from build123d import *

# Parameters (mm, degrees)
BOSS_EXTRUDE1_DEPTH = 2
BOSS_EXTRUDE2_DEPTH = 26
SKETCH2_W           = 20.4
SKETCH2_H           = 20.4
CUT_EXTRUDE1_DEPTH  = 30
CIRPATTERN1_COUNT   = 3
CUT_EXTRUDE2_DEPTH  = 104.592686872
SKETCH4_R           = 2
CUT_EXTRUDE3_DEPTH  = 10
BOSS_EXTRUDE4_START = 26
BOSS_EXTRUDE4_DEPTH = 10
SKETCH5_R           = 2
CUT_EXTRUDE4_DEPTH  = 10
CIRPATTERN2_COUNT   = 3


with BuildPart() as part:
    # Sketch1 → Boss-Extrude1 (new body)
    with BuildSketch(Plane(origin=(0, 0, 0), x_dir=(1, 0, 0), z_dir=(0, 1, 0))):
        Polygon((15, -25.980762114), (30, 0), (15, 25.980762114), (-15, 25.980762114), (-30, 0), (-15, -25.980762114), align=None)
    extrude(amount=BOSS_EXTRUDE1_DEPTH)

    # Sketch1<3> → Boss-Extrude2 (add)
    # profile 1 of 2: a face of its own
    with BuildSketch(Plane(origin=(0, 0, 0), x_dir=(1, 0, 0), z_dir=(0, 1, 0))):
        Polygon((-13, 72.494446501), (-41.141016151, 23.75277675), (-69.282032303, -24.988893001), (-56.282032303, -47.505553499), (0, -47.505553499), (56.282032303, -47.505553499), (69.282032303, -24.988893001), (41.141016151, 23.75277675), (13, 72.494446501), align=None)
        Polygon((-54.549981495, -44.505553499), (-65.817930688, -24.988893001), (-38.54293994, 22.25277675), (-11.267949192, 69.494446501), (11.267949192, 69.494446501), (38.54293994, 22.25277675), (65.817930688, -24.988893001), (54.549981495, -44.505553499), (0, -44.505553499), align=None, mode=Mode.SUBTRACT)
    # profile 2 of 2: a face of its own
    with BuildSketch(Plane(origin=(0, 0, 0), x_dir=(1, 0, 0), z_dir=(0, 1, 0))):
        Polygon((-65.817930688, -24.988893001), (-38.54293994, 22.25277675), (-11.267949192, 69.494446501), (11.267949192, 69.494446501), (38.54293994, 22.25277675), (65.817930688, -24.988893001), (54.549981495, -44.505553499), (0, -44.505553499), (-54.549981495, -44.505553499), align=None)
        Polygon((30, 0), (15, 25.980762114), (-15, 25.980762114), (-30, 0), (-15, -25.980762114), (15, -25.980762114), align=None, mode=Mode.SUBTRACT)
    extrude(amount=BOSS_EXTRUDE2_DEPTH)

    # Sketch2 → Cut-Extrude1 (cut)
    with BuildSketch(Plane(origin=(62.782032303, 0, 36.24722325), x_dir=(0.499999999999999, 0, -0.8660254037844394), z_dir=(0.8660254037844394, 0, 0.499999999999999))):
        with Locations((0, 13)):
            Rectangle(SKETCH2_W, SKETCH2_H)
    cut_extrude1 = extrude(amount=-CUT_EXTRUDE1_DEPTH, mode=Mode.SUBTRACT)

    # CirPattern1: Cut-Extrude1 ×3 about axis
    cirpattern1_axis = Axis((0, 0, 0), (0, 1, 0))
    for i in range(1, CIRPATTERN1_COUNT):
        add(cut_extrude1.rotate(cirpattern1_axis, i * 360 / CIRPATTERN1_COUNT), mode=Mode.SUBTRACT)

    # Sketch3 → Cut-Extrude2 (cut, through all)
    with BuildSketch(Plane(origin=(0, 26, 0), x_dir=(1, 0, 0), z_dir=(0, 1, 0))):
        Polygon((-5.063466521, -1.191342951), (-5.751288694, 0), (-2.875644347, 4.980762114), (-1.5, 4.980762114), (1.5, 4.980762114), (2.875644347, 4.980762114), (5.751288694, 0), (5.063466521, -1.191342951), (3.563466521, -3.789419162), (2.875644347, -4.980762114), (-2.875644347, -4.980762114), (-3.563466521, -3.789419162), align=None)
        Polygon((6.161542732, -5.289419162), (6.911542732, -3.990381057), (7.661542732, -2.691342951), (9.215390309, 0), (7.661542732, 2.691342951), (10.259618943, 4.191342951), (12.679491924, 0), (9.509618943, -5.490381057), (6.339745962, -10.980762114), (1.5, -10.980762114), (1.5, -7.980762114), (4.607695155, -7.980762114), align=None)
        Polygon((-6.339745962, 10.980762114), (0, 10.980762114), (6.339745962, 10.980762114), (8.759618943, 6.789419162), (6.161542732, 5.289419162), (4.607695155, 7.980762114), (1.5, 7.980762114), (0, 7.980762114), (-1.5, 7.980762114), (-4.607695155, 7.980762114), (-6.161542732, 5.289419162), (-8.759618943, 6.789419162), align=None)
        Polygon((-7.661542732, -2.691342951), (-6.911542732, -3.990381057), (-6.161542732, -5.289419162), (-4.607695155, -7.980762114), (-1.5, -7.980762114), (-1.5, -10.980762114), (-6.339745962, -10.980762114), (-9.509618943, -5.490381057), (-12.679491924, 0), (-10.259618943, 4.191342951), (-7.661542732, 2.691342951), (-9.215390309, 0), align=None)
        Polygon((-9.803847577, -16.980762114), (-13.955771366, -9.789419162), (-11.357695155, -8.289419162), (-8.07179677, -13.980762114), (8.07179677, -13.980762114), (11.357695155, -8.289419162), (13.955771366, -9.789419162), (9.803847577, -16.980762114), align=None)
        Polygon((19.607695155, 0), (15.455771366, -7.191342951), (12.857695155, -5.691342951), (16.143593539, 0), (8.07179677, 13.980762114), (1.5, 13.980762114), (1.5, 16.980762114), (9.803847577, 16.980762114), align=None)
        Polygon((-9.803847577, 16.980762114), (-1.5, 16.980762114), (-1.5, 13.980762114), (-8.07179677, 13.980762114), (-16.143593539, 0), (-12.857695155, -5.691342951), (-15.455771366, -7.191342951), (-19.607695155, 0), align=None)
        Polygon((0, 22.980762114), (13.267949192, 22.980762114), (19.151923789, 12.789419162), (16.553847577, 11.289419162), (11.535898385, 19.980762114), (0, 19.980762114), (-11.535898385, 19.980762114), (-16.553847577, 11.289419162), (-19.151923789, 12.789419162), (-13.267949192, 22.980762114), align=None)
        Polygon((-23.07179677, 0), (-17.303847577, -9.990381057), (-11.535898385, -19.980762114), (-1.5, -19.980762114), (-1.5, -22.980762114), (-13.267949192, -22.980762114), (-19.901923789, -11.490381057), (-26.535898385, 0), (-20.651923789, 10.191342951), (-18.053847577, 8.691342951), align=None)
        Polygon((11.535898385, -19.980762114), (17.303847577, -9.990381057), (23.07179677, 0), (18.053847577, 8.691342951), (20.651923789, 10.191342951), (26.535898385, 0), (19.901923789, -11.490381057), (13.267949192, -22.980762114), (1.5, -22.980762114), (1.5, -19.980762114), align=None)
    extrude(amount=-CUT_EXTRUDE2_DEPTH, mode=Mode.SUBTRACT)

    # Sketch4 → Cut-Extrude3 (cut)
    with BuildSketch(Plane.XZ):
        with Locations(Location((0, -64.994446501, 0), (0, 0, 270))):
            Circle(SKETCH4_R)
        with Locations(Location((0, -49.994446501, 0), (0, 0, 270))):
            Circle(SKETCH4_R)
        with Locations(Location((-56.286841774, 32.49722325, 0), (0, 0, 270))):
            Circle(SKETCH4_R)
        with Locations(Location((-43.296460718, 24.99722325, 0), (0, 0, 270))):
            Circle(SKETCH4_R)
        with Locations(Location((56.286841774, 32.49722325, 0), (0, 0, 270))):
            Circle(SKETCH4_R)
        with Locations(Location((43.296460718, 24.99722325, 0), (0, 0, 270))):
            Circle(SKETCH4_R)
    extrude(amount=-CUT_EXTRUDE3_DEPTH, mode=Mode.SUBTRACT)

    # Sketch1<5> → Boss-Extrude4 (add)
    with BuildSketch(Plane(origin=(0, 0, 0), x_dir=(1, 0, 0), z_dir=(0, 1, 0)).offset(BOSS_EXTRUDE4_START)):
        Polygon((-13, 72.494446501), (-41.141016151, 23.75277675), (-69.282032303, -24.988893001), (-56.282032303, -47.505553499), (0, -47.505553499), (56.282032303, -47.505553499), (69.282032303, -24.988893001), (41.141016151, 23.75277675), (13, 72.494446501), align=None)
        Polygon((-54.549981495, -44.505553499), (-65.817930688, -24.988893001), (-38.54293994, 22.25277675), (-11.267949192, 69.494446501), (11.267949192, 69.494446501), (38.54293994, 22.25277675), (65.817930688, -24.988893001), (54.549981495, -44.505553499), (0, -44.505553499), align=None, mode=Mode.SUBTRACT)
    extrude(amount=BOSS_EXTRUDE4_DEPTH)

    # Sketch5 → Cut-Extrude4 (cut)
    with BuildSketch(Plane(origin=(-38.54293994, 0, -22.25277675), x_dir=(0.4999999999999866, 0, -0.8660254037844465), z_dir=(0.8660254037844464, 0, 0.49999999999998657))):
        with Locations((-34.549981495, 31)):
            Circle(SKETCH5_R)
        with Locations((34.549981495, 31)):
            Circle(SKETCH5_R)
    cut_extrude4 = extrude(amount=-CUT_EXTRUDE4_DEPTH, mode=Mode.SUBTRACT)

    # CirPattern2: Cut-Extrude4 ×3 about axis
    cirpattern2_axis = Axis((0, 27.3, 0), (0, -1, 0))
    for i in range(1, CIRPATTERN2_COUNT):
        add(cut_extrude4.rotate(cirpattern2_axis, i * 360 / CIRPATTERN2_COUNT), mode=Mode.SUBTRACT)


solid = part.part
Part model, mm, in its own coordinate system. A direction names the side the tool comes from. Coordinates: 2 decimals unless noted, no trailing zeros. Loops run counter-clockwise (first coordinate to the right, second up) from the corner with the lowest first, then second, coordinate; pieces in that order, holes last. Notation, with made-up numbers: (11, 78.5) -> (53, 78.5) arc R15 ccw to (53, 88.5) -> close; hole circle Ø3 at (86.5, -12). An arc over 180 degrees is marked (long way). Use a Markdown table: item, result. Add a question column.
Item 1: Pull direction Z, two halves, no side cores. Call faces 1 (the cylindrical face through (34.984, 29.048, 45.985)), 2 (the flat face through (16.169, 1.014, -17.956)), 3 (the flat face through (50, 2.8, 29)), 4 (the flat face through (-1, 18, 47.506)): +Z half, -Z half, draft (parallel to the pull), parting line (faces both ways), or undercut.
Item 2: Band-saw the part on B-B on x = 0. Give the number of separate pieces and of enclosed holes in the cut face, plus the area to 3 significant figures.
Item 3: Which spindle directions (+Z, -Z, +X, -X, +Y, -Y) get a long thin tool onto all of the face, cutting with end or side? Do faces 5 (the flat face through (44.9, 12.9, 37.7)), 6 (the flat face through (-11.85, 1.01, 13.44)), 7 (the flat face through (22.395, 13.832, 13.172)), 8 (the flat face through (-50, 23.2, 29)). Say none if no direction does.
Item 4: Band-saw the part on C-C on z = -27.5. Write the cut outline in (x, y), plus the area to 3 significant figures.
Item 5: Band-saw the part on A-A on y = 12. Write the cut outline in (x, z).
Item 6: Flat gauge pins, fed straight in: P1, Ø8, axis at y = 26, z = 34.5, coming from the +X side; P2, Ø1.6, axis at y = 1, z = 9.5, coming from the +X side; P3, Ø10, axis at x = 4.5, z = -55, coming from the +Y side; P4, Ø12, axis at x = 32.5, z = -52, coming from the +Y side. Where does each tip first touch, or does it go through?
Item 7: Probe probe 1 along Y at (x, z) = (44.5, 14); probe 2 along Z at (x, y) = (5.5, 30.5); probe 3 along Z at (x, y) = (3.5, 8.5). List the from-to ranges inside material, lowest first.
Geometry says:
| question | item | result |
|---|---|---|
| 1 | face 1 | draft |
| 1 | face 2 | undercut |
| 1 | face 3 | undercut |
| 1 | face 4 | +Z half |
| 2 | separate pieces | 7 |
| 2 | enclosed holes | 0 |
| 2 | area | 1,260 mm² |
| 3 | face 5 | +X |
| 3 | face 6 | +Y, -Y |
| 3 | face 7 | +Y |
| 3 | face 8 | none |
| 4 | outline | (-38.98, 0) -> (38.98, 0) -> (38.98, 36) -> (35.51, 36) -> (35.51, 26) -> (-35.51, 26) -> (-35.51, 36) -> (-38.98, 36) -> close |
| 4 | area | 2,100 mm² |
| 5 | outline | (-69.28, 24.99) -> (-13, -72.49) -> (-10.2, -72.49) -> (-10.2, -42.49) -> (10.2, -42.49) -> (10.2, -72.49) -> (13, -72.49) -> (69.28, 24.99) -> (67.88, 27.41) -> (41.9, 12.41) -> (31.7, 30.08) -> (57.68, 45.08) -> (56.28, 47.51) -> (-56.28, 47.51) -> (-57.68, 45.08) -> (-31.7, 30.08) -> (-41.9, 12.41) -> (-67.88, 27.41) -> close; hole (-30, 0) -> (-15, -25.98) -> (15, -25.98) -> (30, 0) -> (15, 25.98) -> (-15, 25.98) -> close |
| 6 | P1 | x = 66.1 |
| 6 | P2 | x = 60.8 |
| 6 | P3 | y = 26 |
| 6 | P4 | through |
| 7 | probe 1 | 0 to 2.8, 23.2 to 26 |
| 7 | probe 2 | -72.49 to -69.49, 44.51 to 47.51 |
| 7 | probe 3 | -42.49 to -25.98, 25.98 to 47.51 |
